Verification items for the finished model (mm, model axes). Round coordinates to 2 decimals unless told otherwise and drop trailing zeros. Write each loop counter-clockwise with the first axis right and the second up, starting at its lowest first coordinate (ties: lowest second). Pieces come first, ordered by that corner, then holes. Notation, with made-up numbers: M -5.75,18.5 L 20.25,18.5 A15 cw 20.25,38.5 Z; hole C 0.5,75 d3. An arc over 180 degrees is marked long. One line per item, written item: value. Start each with the question number.
Item 1: Section check A-A, the plane x = 0. Record the cut outline in (y, z), then the cut area to 3 significant figures.
Item 2: Draft check along X on faces 1 (the face through (-7.5, 0, 0)), 2 (the face through (0.46, -0.03, 16.53)), 3 (the face through (0.46, -0.03, -23.47)), 4 (the face through (0, 0, 27)). Enter one of: +X half, -X half, draft (parallel to the pull), parting line (faces both ways), or undercut.
Item 3: Section check C-C, the plane y = -1.2. Record the cut outline in (x, z).
Item 4: Thickness scan on probe 1 along Z at (x, y) = (0, 0.25); probe 2 along Z at (x, y) = (-3, -0.3); probe 3 along X at (y, z) = (-0.65, 18.5). Record the ranges inside material, lowest first. Write a range as from..to.
Item 5: Section check D-D, the plane z = 22. Record the cut outline in (x, y), then the cut area to 3 significant figures.
Item 6: Section check B-B, the plane z = -20. Record the cut outline in (x, y), then the cut area to 3 significant figures.
Autodesk Inventor part; units mm, degrees
ref_plane "YZ Plane" through (0, 0, 0) normal (1, 0, 0) x (0, 1, 0)
ref_plane "XZ Plane" through (0, 0, 0) normal (0, 1, 0) x (-1, 0, 0)
ref_plane "XY Plane" through (0, 0, 0) normal (0, 0, 1) x (1, 0, 0)
sketch "Sketch1" plane through (0, 0, 0) normal (0, 1, 0) x (-1, 0, 0)
  line L0 (-7.5, 27) -> (7.5, 27)
  line L1 (7.5, 27) -> (7.5, -27)
  line L2 (7.5, -27) -> (-7.5, -27)
  line L3 (-7.5, -27) -> (-7.5, 27)
  line L4 (-7.5, 27) -> (7.5, -27) construction
  line L5 (7.5, 27) -> (-7.5, -27) construction
  circle A0 centre (0, -20) radius 3.5
  circle A1 centre (0, 20) radius 3.5
  line L6 (7.5, 0) -> (0, 0)
  point P0 (0, 0)
  dimension "d0" = 7
  dimension "d1" = 15
  dimension "d2" = 54
  dimension "d3" = 40
extrude "Extrusion1" add sketch "Sketch1" along normal mid plane 4
properties part number "Планка" material "Stainless Steel"
Response values:
1. outline: M -2,-27 L 2,-27 L 2,-23.5 L -2,-23.5 Z; M -2,-16.5 L 2,-16.5 L 2,16.5 L -2,16.5 Z; M -2,23.5 L 2,23.5 L 2,27 L -2,27 Z
1. area: 160 mm2
2. face 1: -X half
2. face 2: undercut
2. face 3: undercut
2. face 4: draft
3. outline: M -7.5,-27 L 7.5,-27 L 7.5,27 L -7.5,27 Z; hole C 0,-20 d7; hole C 0,20 d7
4. probe 1: z = -27..-23.5, -16.5..16.5, 23.5..27
4. probe 2: z = -27..-21.8, -18.2..18.2, 21.8..27
4. probe 3: x = -7.5..-3.16, 3.16..7.5
5. outline: M -7.5,-2 L -2.87,-2 L -2.87,2 L -7.5,2 Z; M 2.87,-2 L 7.5,-2 L 7.5,2 L 2.87,2 Z
5. area: 37.0 mm2
6. outline: M -7.5,-2 L -3.5,-2 L -3.5,2 L -7.5,2 Z; M 3.5,-2 L 7.5,-2 L 7.5,2 L 3.5,2 Z
6. area: 32.0 mm2
